from build123d import *

# Parameters (mm, degrees)
F0_W     = 127
F0_H     = 76.2
F1_DEPTH = 50.8
F2_R     = 5.08
F3_W     = 7
F3_H     = 14.3
F4_DEPTH = 16.4
F6_DEPTH = 16.4084


with BuildPart() as f1:
    # F0 (on Front) → F1 (new body)
    with BuildSketch(Plane.XZ):
        Rectangle(F0_W, F0_H)
    extrude(amount=F1_DEPTH)

    # F2
    f2_edges = [f1.edges().sort_by_distance(p)[0] for p in [
        (0, -50.8, 38.1),
        (0, 0, 38.1),
        (0, 0, -38.1),
        (0, -50.8, -38.1),
    ]]
    fillet(f2_edges, radius=F2_R)

    # F3 (on face) → F4 (cut)
    with BuildSketch(Plane.YZ.offset(63.5)):
        with Locations((-42.22, 24.25)):
            Rectangle(F3_W, F3_H)
    extrude(amount=-F4_DEPTH, mode=Mode.SUBTRACT)

    # F5 (on face) → F6 (cut)
    with BuildSketch(Plane.YZ.offset(63.5)):
        with BuildLine():
            Line((-24.988418, 31.4), (-27.988418, 31.4))
            ThreePointArc((-27.988418, 31.4), (-29.402631, 30.814213), (-29.988418, 29.4))
            Line((-29.988418, 29.4), (-29.988418, 19.1))
            ThreePointArc((-29.988418, 19.1), (-29.402631, 17.685786), (-27.988418, 17.1))
            Line((-27.988418, 17.1), (-24.988418, 17.1))
            ThreePointArc((-24.988418, 17.1), (-23.574204, 17.685786), (-22.988418, 19.1))
            Line((-22.988418, 19.1), (-22.988418, 29.4))
            ThreePointArc((-22.988418, 29.4), (-23.574204, 30.814213), (-24.988418, 31.4))
        make_face()
    extrude(amount=-F6_DEPTH, mode=Mode.SUBTRACT)


solid = f1.part
The model under review builds one solid part; all positions refer to its coordinate system, in mm. A direction names the side the tool comes from. Give positions to 0.01 mm unless a question says otherwise; leave off trailing zeros. Write each loop counter-clockwise with the first axis right and the second up, starting at its lowest first coordinate (ties: lowest second). Pieces come first, ordered by that corner, then holes.
1. Draft analysis for pull direction Z (two halves, no side actions). For faces 3 (the flat face through (55, -26, 31.4)), 4 (the flat face through (-1, -25, 38.1)), 5 (the flat face through (-63.5, -25, -1)), 6 (the flat face through (-1, -25, -38.1)), state which applies: +Z half, -Z half, draft (parallel to the pull), parting line (faces both ways), or undercut.
2. For P1, Ø2, axis at y = -25.5, z = 25, coming from the +X side, flat-tipped, find the tip position at first contact; note if it passes through.
3. Add section B-B, the plane y = -40. Write out the cut boundary in (x, z), plus the area to 3 significant figures.
4. Add section A-A, the plane z = 20.5. Write out the cut boundary in (x, y), plus the area to 3 significant figures.
5. Wall thickness on L1, parallel to X at y = -42.5, z = 30.5; L2, parallel to Z at x = -56.5, y = -3; L3, parallel to Y at x = -8.5, z = 34.5: over which ranges is each line inside the solid? List them lowest first.
6. Tool access review of faces 1 (the flat face through (55, -42, 17.1)), 2 (the flat face through (63.5, -25, -1)): name each direction out of +Z, -Z, +X, -X, +Y, -Y from which nothing blocks a thin tool from reaching the whole face with its end or side.
Worked answers:
1. face 3: undercut
1. face 4: +Z half
1. face 5: draft
1. face 6: -Z half
2. P1: stops at x = 47.09
3. outline: (-63.5, -38.1) - (63.5, -38.1) - (63.5, 17.1) - (47.1, 17.1) - (47.1, 31.4) - (63.5, 31.4) - (63.5, 38.1) - (-63.5, 38.1) - close
3. area: 9,440 mm2
4. outline: (-63.5, -50.8) - (63.5, -50.8) - (63.5, -45.72) - (47.1, -45.72) - (47.1, -38.72) - (63.5, -38.72) - (63.5, -29.99) - (47.09, -29.99) - (47.09, -22.99) - (63.5, -22.99) - (63.5, 0) - (-63.5, 0) - close
4. area: 6,220 mm2
5. L1: x = -63.5 to 47.1
5. L2: z = -37.65 to 37.65
5. L3: y = -50.58 to -0.22
6. face 1: +X
6. face 2: +Z, -Z, +X, +Y, -Y
